from build123d import *

# Parameters (mm, degrees)
BOSS_EXTRUDE1_DEPTH            = 5
M5_CLEARANCE_HOLE1_D           = 5.5
M5_CLEARANCE_HOLE1_CSINK_D     = 5.55
M5_CLEARANCE_HOLE1_CSINK_ANGLE = 90


with BuildPart() as part:
    # Sketch1 → Boss-Extrude1 (new body)
    with BuildSketch(Plane.XY):
        with BuildLine():
            Line((1, 0), (39, 0))
            ThreePointArc((39, 0), (39.707106781, 0.292893219), (40, 1))
            Line((40, 1), (40, 19))
            ThreePointArc((40, 19), (39.707106781, 19.707106781), (39, 20))
            Line((39, 20), (21, 20))
            ThreePointArc((21, 20), (20.292893219, 20.292893219), (20, 21))
            Line((20, 21), (20, 39))
            ThreePointArc((20, 39), (19.707106781, 39.707106781), (19, 40))
            Line((19, 40), (1, 40))
            ThreePointArc((1, 40), (0.292893219, 39.707106781), (0, 39))
            Line((0, 39), (0, 1))
            ThreePointArc((0, 1), (0.292893219, 0.292893219), (1, 0))
        make_face()
    extrude(amount=BOSS_EXTRUDE1_DEPTH)

    # M5 Clearance Hole1 (through all)
    with Locations(Plane.XY.offset(5)):
        with Locations((10, 30), (10, 10), (30, 10)):
            CounterSinkHole(M5_CLEARANCE_HOLE1_D / 2, M5_CLEARANCE_HOLE1_CSINK_D / 2, counter_sink_angle=M5_CLEARANCE_HOLE1_CSINK_ANGLE)


solid = part.part
Input: part model. Units: mm. Frame: model coordinates. A direction names the side the tool comes from. Coordinates: 2 decimals unless noted, no trailing zeros. Loops run counter-clockwise (first coordinate to the right, second up) from the corner with the lowest first, then second, coordinate; pieces in that order, holes last.
Q1. Cut plane C-C (x = 30). Output: boundary loops of the cut face in (y, z) (3 decimals).
Q2. Set-up query: faces 1 (the face through (0, 20, 2)), 2 (the face through (20, 30, 2)). Return all of +Z, -Z, +X, -X, +Y, -Y with unobstructed straight access to the full face (end or side cutting, diameter ignored); none if empty.
Q3. Cut plane A-A (y = 10). Output: boundary loops of the cut face in (x, z) (3 decimals).
Q4. Material intervals for line 1 (Y direction, x = 10, z = 3.75); line 2 (X direction, y = 7.5, z = 0.25), sorted ascending.
Q5. Contact query for a flat-ended pin moving along its axis: pin 1 (1 mm diameter, centred on x = 27.5, z = 1.5, fed in from +Y). Output: stop coordinate, or through.
Q6. Cut plane D-D (z = 0.5). Output: boundary loops of the cut face in (x, y), then the cut area to 3 significant figures.
Working result:
1. outline: (0, 0) - (7.25, 0) - (7.25, 4.975) - (7.225, 5) - (0, 5) - close; (12.75, 0) - (20, 0) - (20, 5) - (12.775, 5) - (12.75, 4.975) - close
2. face 1: +Z, -Z, -X, +Y, -Y
2. face 2: +Z, -Z, +X, +Y
3. outline: (0, 0) - (7.25, 0) - (7.25, 4.975) - (7.225, 5) - (0, 5) - close; (12.75, 0) - (27.25, 0) - (27.25, 4.975) - (27.225, 5) - (12.775, 5) - (12.75, 4.975) - close; (32.75, 0) - (40, 0) - (40, 5) - (32.775, 5) - (32.75, 4.975) - close
4. line 1: y = 0 to 7.25, 12.75 to 27.25, 32.75 to 40
4. line 2: x = 0 to 8.85, 11.15 to 28.85, 31.15 to 40
5. pin 1: stops at y = 20
6. outline: (0, 1) arc R1 ccw to (1, 0) - (39, 0) arc R1 ccw to (40, 1) - (40, 19) arc R1 ccw to (39, 20) - (21, 20) arc R1 cw to (20, 21) - (20, 39) arc R1 ccw to (19, 40) - (1, 40) arc R1 ccw to (0, 39) - close; hole circle Ø5.5 at (10, 10); hole circle Ø5.5 at (10, 30); hole circle Ø5.5 at (30, 10)
6. area: 1,130 mm2
